Could you check a few things on this drawing? It's one solid part, dimensions in mm from its lowest x, y, z. A direction names the side the tool comes from. Give positions to 0.01 mm unless a question says otherwise; leave off trailing zeros. Order: outer loops, then holes, each group sorted by start corner. A loop starts at its lowest first (then second) coordinate and runs counter-clockwise, first axis right, second up. Notation, with made-up numbers: (76.5, -7) - (96.5, -7) arc R17 ccw to (96.5, 26) - close; hole circle Ø6 at (-36.75, 44). An arc over 180 degrees is marked (long way). Return JSON: item names as keys, results as strings.
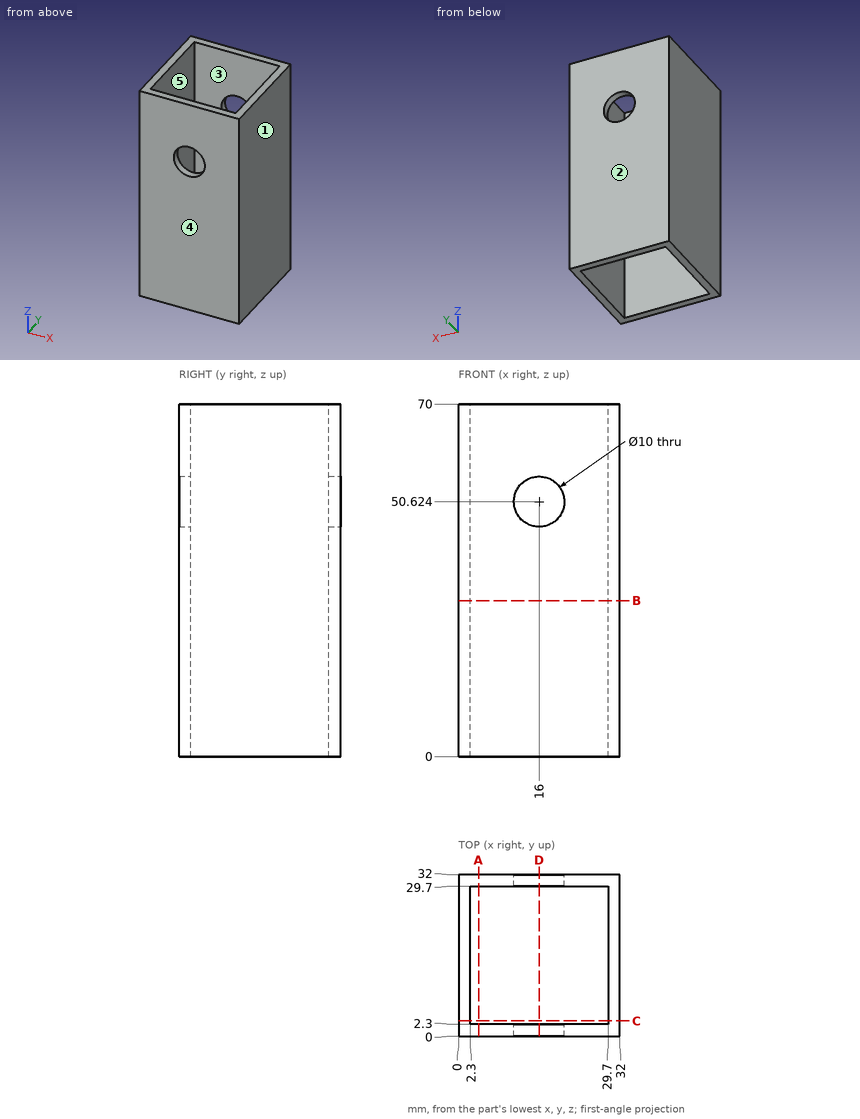
1. For pin 1 Ø13.5 at (y, z) = (17, 20) entering from -X, with a flat end and sliding along its axis, tell me the tip position at first contact or that it passes through.
Checks:
{"pin 1": "x = 0"}
2. Suppose I cut it at B-B (z = 31). List the corners of the cut face in (x, y) for me, plus the area to 3 significant figures.
Checks:
{"outline": "(0, 0) - (32, 0) - (32, 32) - (0, 32) - close; hole (2.3, 2.3) - (29.7, 2.3) - (29.7, 29.7) - (2.3, 29.7) - close", "area": "273 mm^2"}
3. Suppose I cut it at D-D (x = 16). List the corners of the cut face in (y, z) for me.
Checks:
{"outline": "(0, 0) - (2.3, 0) - (2.3, 45.62) - (0, 45.62) - close; (0, 55.62) - (2.3, 55.62) - (2.3, 70) - (0, 70) - close; (29.7, 0) - (32, 0) - (32, 45.62) - (29.7, 45.62) - close; (29.7, 55.62) - (32, 55.62) - (32, 70) - (29.7, 70) - close"}
4. On a 3-axis mill with a long thin cutter (end or side, diameter ignored), from which of +Z, -Z, +X, -X, +Y, -Y can I reach the whole of each face in a straight line? I mean the marked faces 4 and 5. Say none if no direction works.
Checks:
{"face 4": "+Z, -Z, +X, -X, -Y", "face 5": "+Z, -Z"}
5. If I drill on L1, parallel to Y at x = 15.5, z = 29; L2, parallel to Z at x = 16, y = 30, over which ranges is the centre line in solid material (lowest first)? Write a range as [from, to].
Checks:
{"L1": "[0, 2.3], [29.7, 32]", "L2": "[0, 45.62], [55.62, 70]"}
6. Suppose I cut it at A-A (x = 4). List the corners of the cut face in (y, z) for me, plus the area to 3 significant figures.
Checks:
{"outline": "(0, 0) - (2.3, 0) - (2.3, 70) - (0, 70) - close; (29.7, 0) - (32, 0) - (32, 70) - (29.7, 70) - close", "area": "322 mm^2"}
7. Thinking about a two-plate mould opening in X: for the marked faces 1, 2 and 3, which applies, +X half, -X half, draft (parallel to the pull), parting line (faces both ways), or undercut?
Checks:
{"face 1": "+X half", "face 2": "draft", "face 3": "undercut"}
